Part model, mm, in its own coordinate system. Face numbers are marked on the shaded views. A direction names the side the tool comes from. Round coordinates to 2 decimals unless told otherwise and drop trailing zeros. Write each loop counter-clockwise with the first axis right and the second up, starting at its lowest first coordinate (ties: lowest second). Pieces come first, ordered by that corner, then holes. Notation, with made-up numbers: (39.25, 82) -> (92.25, 82) arc R22 ccw to (92.25, 112) -> close; hole circle Ø2 at (-25, -2). An arc over 180 degrees is marked (long way). Return JSON: item names as keys, results as strings. Group by question number.
(1) Saw through at A-A (y = 4). List the corners of the cut face in (x, z), plus the area to 3 significant figures.
(2) Tool access for the marked faces 5, 6 and 7: list every direction of +Z, -Z, +X, -X, +Y, -Y with a clear straight run to the whole face (end or side of a thin tool).
(3) Saw through at D-D (y = 13.25). List the corners of the cut face in (x, z).
(4) Saw through at C-C (z = -1.5). List the corners of the cut face in (x, y).
(5) Drop flat-ended pins along their axis: pin 1 Ø10 at (y, z) = (16, -2) entering from -X; pin 2 Ø8 at (x, z) = (-39.5, 8.5) entering from -Y; pin 3 Ø2 at (x, z) = (2.5, -4.5) entering from +Y; pin 4 Ø7.5 at (x, z) = (45, 0) entering from -Y. Give the stop position or say it passes through.
(6) Drill centre lines: L1, parallel to Z at x = 20.5, y = 15.5; L2, parallel to X at y = 9.75, z = -6; L3, parallel to X at y = 4.75, z = -18.5. Where is each one in solid material? Low to high. Write a range as from..to.
(7) Saw through at B-B (x = 42.5). List the corners of the cut face in (y, z).
(8) Mould opens along Z. For the marked faces 1, 2, 3 and 4 say: +Z half, -Z half, draft (parallel to the pull), parting line (faces both ways), or undercut.
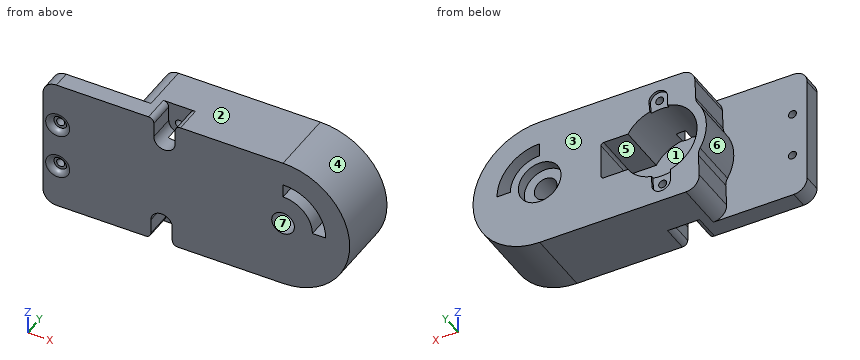
from build123d import *

# Parameters (mm, degrees)
BOSS_EXTRUDE1_DEPTH = 25
SKETCH2_R           = 14
CUT_EXTRUDE1_DEPTH  = 19
CUT_EXTRUDE2_DEPTH  = 1
SKETCH4_R           = 1.5
CUT_EXTRUDE3_DEPTH  = 79.108898341
SKETCH5_R           = 1.5
CUT_EXTRUDE4_DEPTH  = 79.108898341
CUT_EXTRUDE7_DEPTH  = 19
FILLET1_R           = 1
CUT_EXTRUDE8_DEPTH  = 18.4
FILLET2_R           = 5
SKETCH8_R           = 1.5
CUT_EXTRUDE9_DEPTH  = 77.573885888
SKETCH9_R           = 2.5
CUT_EXTRUDE10_DEPTH = 2
FILLET3_R           = 2
CUT_EXTRUDE11_DEPTH = 10
FILLET4_R           = 2
SKETCH11_R          = 8
CUT_EXTRUDE12_DEPTH = 4
SKETCH12_R          = 4.25
CUT_EXTRUDE13_DEPTH = 78.239886096
CUT_EXTRUDE16_DEPTH = 25


with BuildPart() as part:
    # Sketch1 → Boss-Extrude1 (new body)
    with BuildSketch(Plane(origin=(0, 0, 0), x_dir=(1, 0, 0), z_dir=(0, 1, 0))):
        with BuildLine():
            Line((-45, 25), (45, 25))
            ThreePointArc((45, 25), (70, 0), (45, -25))
            Line((45, -25), (-45, -25))
            Line((-45, -25), (-45, 25))
        make_face()
    extrude(amount=BOSS_EXTRUDE1_DEPTH)

    # Sketch2 → Cut-Extrude1 (cut)
    with BuildSketch(Plane(origin=(0, 25, 0), x_dir=(1, 0, 0), z_dir=(0, 1, 0))):
        with Locations(Location((0, 0, 0), (0, 0, 270))):
            Circle(SKETCH2_R)
    extrude(amount=-CUT_EXTRUDE1_DEPTH, mode=Mode.SUBTRACT)

    # Sketch3 → Cut-Extrude2 (cut)
    with BuildSketch(Plane(origin=(0, 25, 0), x_dir=(1, 0, 0), z_dir=(0, 1, 0))):
        with BuildLine():
            ThreePointArc((2.953843371, 17.491475436), (-0.546156629, 20.991475436), (-4.046156629, 17.491475436))
            Line((-4.046156629, 17.491475436), (-4.046156629, 13.402560074))
            ThreePointArc((-4.046156629, 13.402560074), (-0.522473122, 13.990247383), (3.035229041, 13.667018134))
            Line((3.035229041, 13.667018134), (2.953843371, 17.491475436))
        make_face()
        with BuildLine():
            Line((-2.953843371, -13.684838667), (-2.953843371, -17.491475436))
            ThreePointArc((-2.953843371, -17.491475436), (0.546156629, -20.991475436), (4.046156629, -17.491475436))
            Line((4.046156629, -17.491475436), (3.686093385, -13.506025158))
            ThreePointArc((3.686093385, -13.506025158), (0.376883388, -13.994926185), (-2.953843371, -13.684838667))
        make_face()
    extrude(amount=-CUT_EXTRUDE2_DEPTH, mode=Mode.SUBTRACT)

    # Sketch4 → Cut-Extrude3 (cut, through all)
    with BuildSketch(Plane(origin=(0, 24, 0), x_dir=(1, 0, 0), z_dir=(0, 1, 0))):
        with Locations(Location((-0.546156629, 17.491475436, 0), (0, 0, 270))):
            Circle(SKETCH4_R)
    extrude(amount=-CUT_EXTRUDE3_DEPTH, mode=Mode.SUBTRACT)

    # Sketch5 → Cut-Extrude4 (cut, through all)
    with BuildSketch(Plane(origin=(0, 24, 0), x_dir=(1, 0, 0), z_dir=(0, 1, 0))):
        with Locations(Location((0.546156629, -17.491475436, 0), (0, 0, 270))):
            Circle(SKETCH5_R)
    extrude(amount=-CUT_EXTRUDE4_DEPTH, mode=Mode.SUBTRACT)

    # Sketch6 → Cut-Extrude7 (cut)
    with BuildSketch(Plane(origin=(0, 25, 0), x_dir=(1, 0, 0), z_dir=(0, 1, 0))):
        with BuildLine():
            Line((22, 7.35), (22, -7.35))
            Line((22, -7.35), (11.915431171, -7.35))
            Line((11.915431171, -7.35), (11.920287143, -7.342121929))
            ThreePointArc((11.920287143, -7.342121929), (13.999999235, 0.004627215), (11.915431171, 7.35))
            Line((11.915431171, 7.35), (22, 7.35))
        make_face()
    extrude(amount=-CUT_EXTRUDE7_DEPTH, mode=Mode.SUBTRACT)

    # Fillet1
    fillet1_edges = [part.edges().sort_by_distance(p)[0] for p in [
        (22, 15.5, 7.35),
        (22, 15.5, -7.35),
    ]]
    fillet(fillet1_edges, radius=FILLET1_R)

    # Sketch7 → Cut-Extrude8 (cut)
    with BuildSketch(Plane(origin=(0, 25, 0), x_dir=(1, 0, 0), z_dir=(0, 1, 0))):
        with BuildLine():
            Line((-14.411704874, 9.927374408), (-15.019516237, 25))
            Line((-15.019516237, 25), (-45, 25))
            Line((-45, 25), (-45, -25))
            Line((-45, -25), (-13.003240573, -25))
            Line((-13.003240573, -25), (-13.565556796, -11.055571845))
            ThreePointArc((-13.565556796, -11.055571845), (-17.485788544, -0.705123398), (-14.411704874, 9.927374408))
        make_face()
    extrude(amount=-CUT_EXTRUDE8_DEPTH, mode=Mode.SUBTRACT)

    # Fillet2
    fillet2_edges = [part.edges().sort_by_distance(p)[0] for p in [
        (-45, 3.3, 25),
        (-45, 3.3, -25),
        (-14.411704874, 15.8, -9.927374408),
        (-13.565556796, 15.8, 11.055571845),
        (-13.003240573, 15.8, 25),
        (-15.019516237, 15.8, -25),
    ]]
    fillet(fillet2_edges, radius=FILLET2_R)

    # Sketch8 → Cut-Extrude9 (cut, through all)
    with BuildSketch(Plane(origin=(0, 6.6, 0), x_dir=(1, 0, 0), z_dir=(0, 1, 0))):
        with Locations(Location((-39.5, 8.5, 0), (0, 0, 270))):
            Circle(SKETCH8_R)
        with Locations(Location((-39.5, -8.5, 0), (0, 0, 270))):
            Circle(SKETCH8_R)
    extrude(amount=-CUT_EXTRUDE9_DEPTH, mode=Mode.SUBTRACT)

    # Sketch9 → Cut-Extrude10 (cut)
    with BuildSketch(Plane.XZ):
        with Locations(Location((-39.5, 8.5, 0), (0, 0, 270))):
            Circle(SKETCH9_R)
        with Locations(Location((-39.5, -8.5, 0), (0, 0, 270))):
            Circle(SKETCH9_R)
    extrude(amount=-CUT_EXTRUDE10_DEPTH, mode=Mode.SUBTRACT)

    # Fillet3
    fillet3_edges = [part.edges().sort_by_distance(p)[0] for p in [
        (-39.5, 0, 11),
        (-39.5, 0, -6),
    ]]
    fillet(fillet3_edges, radius=FILLET3_R - 0.0001)  # a hair under: the kernel refuses the full size

    # Sketch10 → Cut-Extrude11 (cut)
    with BuildSketch(Plane.XZ):
        with BuildLine():
            Line((-3.453843371, 17.491475436), (-3.453843371, 25))
            Line((-3.453843371, 25), (4.546156629, 25))
            Line((4.546156629, 25), (4.546156629, 17.491475436))
            ThreePointArc((4.546156629, 17.491475436), (0.546156629, 13.491475436), (-3.453843371, 17.491475436))
        make_face()
        with BuildLine():
            Line((-4.546156629, -17.491475436), (-4.546156629, -25))
            Line((-4.546156629, -25), (3.453843371, -25))
            Line((3.453843371, -25), (3.453843371, -17.491475436))
            ThreePointArc((3.453843371, -17.491475436), (-0.546156629, -13.491475436), (-4.546156629, -17.491475436))
        make_face()
    extrude(amount=-CUT_EXTRUDE11_DEPTH, mode=Mode.SUBTRACT)

    # Fillet4
    fillet4_edges = [part.edges().sort_by_distance(p)[0] for p in [
        (-3.453843371, 5, 25),
        (4.546156629, 5, 25),
        (3.453843371, 5, -25),
        (-4.546156629, 5, -25),
    ]]
    fillet(fillet4_edges, radius=FILLET4_R)

    # Sketch11 → Cut-Extrude12 (cut)
    with BuildSketch(Plane(origin=(0, 25, 0), x_dir=(1, 0, 0), z_dir=(0, 1, 0))):
        with Locations(Location((45, 0, 0), (0, 0, 270))):
            Circle(SKETCH11_R)
    extrude(amount=-CUT_EXTRUDE12_DEPTH, mode=Mode.SUBTRACT)

    # Sketch12 → Cut-Extrude13 (cut, through all)
    with BuildSketch(Plane(origin=(0, 21, 0), x_dir=(1, 0, 0), z_dir=(0, 1, 0))):
        with Locations(Location((45, 0, 0), (0, 0, 270))):
            Circle(SKETCH12_R)
    extrude(amount=-CUT_EXTRUDE13_DEPTH, mode=Mode.SUBTRACT)

    # Sketch19 → Cut-Extrude16 (cut)
    with BuildSketch(Plane.XZ):
        with BuildLine():
            Line((45, 11), (45, 16))
            ThreePointArc((45, 16), (56.313708499, 11.313708499), (61, 0))
            Line((61, 0), (56, 0))
            ThreePointArc((56, 0), (52.778174593, 7.778174593), (45, 11))
        make_face()
    extrude(amount=-CUT_EXTRUDE16_DEPTH, mode=Mode.SUBTRACT)


solid = part.part
Computed values:
{
 "1": {"outline": "(-45, -20) arc R5 ccw to (-40, -25) -> (-6.55, -25) arc R2 ccw to (-4.55, -23) -> (-4.55, -17.49) arc R4 cw to (3.45, -17.49) -> (3.45, -23) arc R2 ccw to (5.45, -25) -> (45, -25) arc R25 ccw to (45, 25) -> (6.55, 25) arc R2 ccw to (4.55, 23) -> (4.55, 17.49) arc R4 cw to (-3.45, 17.49) -> (-3.45, 23) arc R2 ccw to (-5.45, 25) -> (-40, 25) arc R5 ccw to (-45, 20) -> close; hole circle Ø3 at (-39.5, -8.5); hole circle Ø3 at (-39.5, 8.5); hole circle Ø8.5 at (45, 0); hole (45, 11) arc R11 cw to (56, 0) -> (61, 0) arc R16 ccw to (45, 16) -> close", "area": "5,120 mm2"},
 "2": {"face 5": "+Y", "face 6": "-X, +Y", "face 7": "+Y, -Y"},
 "3": {"outline": "(-15.14, -8.77) arc R5 cw to (-14.47, -11.48) -> (-14.81, -19.8) arc R5 ccw to (-9.81, -25) -> (45, -25) arc R25 ccw to (45, 25) -> (-8.2, 25) arc R5 ccw to (-13.2, 20.2) -> (-13.5, 12.61) arc R5 cw to (-14.39, 9.96) arc R17.5 ccw to start; hole circle Ø3 at (-0.55, -17.49); hole circle Ø3 at (0.55, 17.49); hole (11.92, -7.35) -> (21, -7.35) arc R1 ccw to (22, -6.35) -> (22, 6.35) arc R1 ccw to (21, 7.35) -> (11.92, 7.35) arc R14 ccw (long way) to start; hole circle Ø8.5 at (45, 0); hole (45, 11) arc R11 cw to (56, 0) -> (61, 0) arc R16 ccw to (45, 16) -> close"},
 "4": {"outline": "(-45, 0) -> (41.02, 0) -> (41.02, 21) -> (37.14, 21) -> (37.14, 25) -> (22, 25) -> (22, 6) -> (-13.92, 6) -> (-13.92, 25) -> (-17.44, 25) -> (-17.44, 6.6) -> (-45, 6.6) -> close; (48.98, 0) -> (69.95, 0) -> (69.95, 25) -> (52.86, 25) -> (52.86, 21) -> (48.98, 21) -> close"},
 "5": {"pin 1": "x = -17.5", "pin 2": "y = 0.06", "pin 3": "y = 6", "pin 4": "through"},
 "6": {"L1": "-25..-7.35, 7.35..25", "L2": "-16.44..-12.65, 22..69.27", "L3": "-45..-4.55, 3.45..61.82"},
 "7": {"outline": "(0, -25) -> (25, -25) -> (25, -7.6) -> (21, -7.6) -> (21, -3.44) -> (0, -3.44) -> close; (0, 3.44) -> (21, 3.44) -> (21, 7.6) -> (25, 7.6) -> (25, 25) -> (0, 25) -> close"},
 "8": {"face 1": "undercut", "face 2": "+Z half", "face 3": "draft", "face 4": "parting line"}
}
